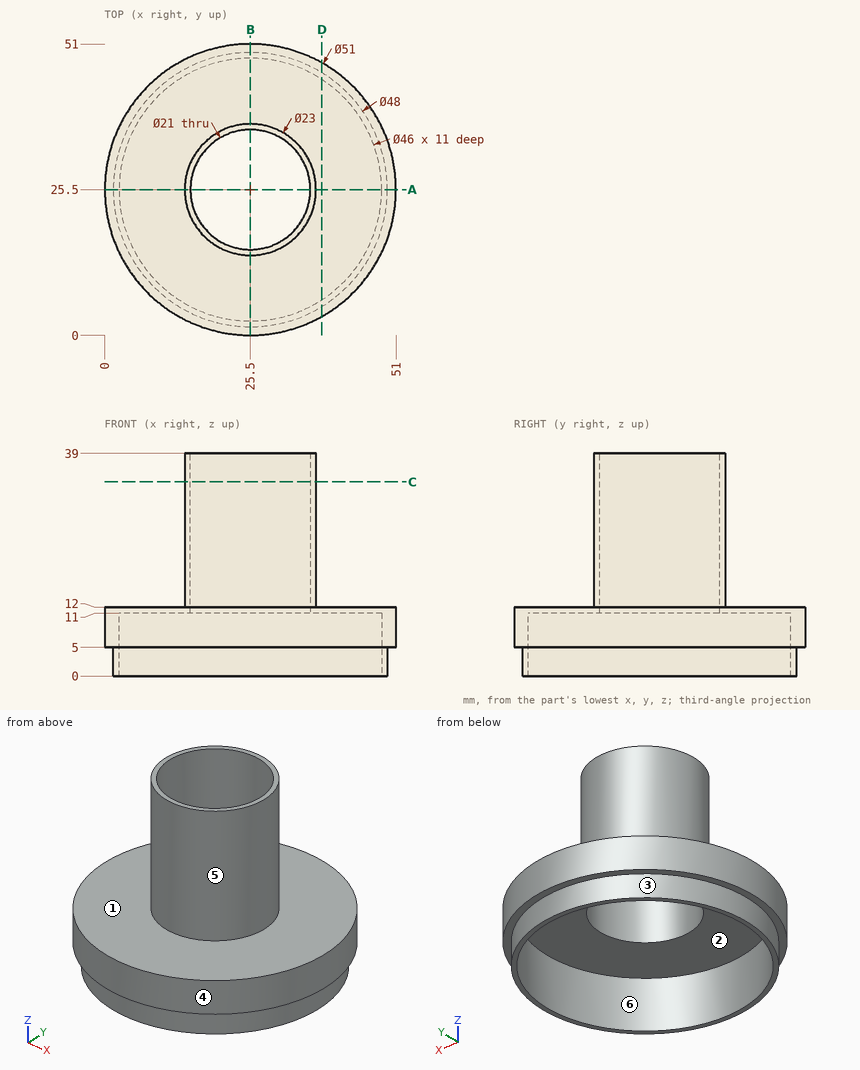
Answer from the drawing. Dimensions are ordinates in mm from the lowest x, y and z of the part. A direction names the side the tool comes from. Round coordinates to 2 decimals unless told otherwise and drop trailing zeros. Write each loop counter-clockwise with the first axis right and the second up, starting at its lowest first coordinate (ties: lowest second). Pieces come first, ordered by that corner, then holes. Notation, with made-up numbers: M 71,84.25 L 81,84.25 A13 ccw 81,94.25 Z; hole C 1,46.5 d2. An arc over 180 degrees is marked long. Write each question's results on one line, items separated by ' | '. Start each with the question number.
Item 1: A cutting plane is placed at D-D on x = 38. Write down the section's boundary in (y, z), and give its area (3 significant figures).
Item 2: A cutting plane is placed at A-A on y = 25.5. Write down the section's boundary in (x, z), and give its area (3 significant figures).
Item 3: For a pull along Y with two mould halves and no side action, classify the marked faces 1, 2 and 3 as pulls with the +Y half, pulls with the -Y half, needs draft (parallel to the pull), parting line crosses it, or undercut.
Item 4: Flat-ended cylindrical pins translate along their axes: pin 1 Ø2 at (x, y) = (33.5, 43.5) entering from +Z; pin 2 Ø3 at (x, y) = (28.5, 12) entering from -Z; pin 3 Ø8 at (x, z) = (17, 30.5) entering from +Y; pin 4 Ø3 at (x, y) = (45.5, 35) entering from -Z. Find the tip coordinate at first contact, or state that the pin passes through.
Item 5: Straight lines are drawn through the part: L1, parallel to X at y = 25, z = 28; L2, parallel to Y at x = 25.5, z = 7.5; L3, parallel to Y at x = 25.5, z = 4.5. For each, find the intervals that lie inside material, in ascending order. Write a range as [from, to].
Item 6: A cutting plane is placed at C-C on z = 34. Write down the section's boundary in (x, y), and give its area (3 significant figures).
Item 7: For the marked faces 4, 5 and 6, determine the directions among +Z, -Z, +X, -X, +Y, -Y from which every point of the face is accessible in a straight line to the end or side of a thin tool.
Check sheet entries:
1) outline: M 3.27,5 L 5.01,5 L 5.01,0 L 6.19,0 L 6.19,11 L 44.81,11 L 44.81,0 L 45.99,0 L 45.99,5 L 47.73,5 L 47.73,12 L 3.27,12 Z | area: 91.3 mm²
2) outline: M 0,5 L 1.5,5 L 1.5,0 L 2.5,0 L 2.5,11 L 15,11 L 15,39 L 14,39 L 14,12 L 0,12 Z; M 36,11 L 48.5,11 L 48.5,0 L 49.5,0 L 49.5,5 L 51,5 L 51,12 L 37,12 L 37,39 L 36,39 Z | area: 124 mm²
3) face 1: needs draft | face 2: undercut | face 3: parting line crosses it
4) pin 1: z = 12 | pin 2: z = 11 | pin 3: y = 36.08 | pin 4: z = 0
5) L1: [14.01, 15.01], [35.99, 36.99] | L2: [0, 2.5], [48.5, 51] | L3: [1.5, 2.5], [48.5, 49.5]
6) outline: C 25.5,25.5 d23; hole C 25.5,25.5 d21 | area: 69.1 mm²
7) face 4: +Z, -Z | face 5: +Z | face 6: -Z
